from build123d import *

# Parameters (mm, degrees)
F0_W             = 150
F0_H             = 80
F1_DEPTH         = 8
F2_SIZE          = 2.5
F4_D             = 4.4
F4_COPIES_COUNT  = 4
F4_COPIES2_COUNT = 2
F4_COPIES2_PITCH = 104.737768
F4_COPIES3_COUNT = 2
F4_COPIES3_PITCH = 92.195445
F4_COPIES4_COUNT = 2
F4_COPIES4_PITCH = 67.720012
F5_D             = 6.5
F6_D             = 5.5
F7_D             = 29


# Not quite as in the source:
# - a pattern or mirror of a feature is missing from the dataset's text; its kind, count and spacing are read off the source's solid


with BuildPart() as f1:
    # F0 (on Front) → F1 (new body)
    with BuildSketch(Plane.XZ):
        Rectangle(F0_W, F0_H)
    extrude(amount=F1_DEPTH)

    # F2
    f2_edges = [f1.edges().sort_by_distance(p)[0] for p in [
        (75, -4, 40),
        (75, -4, -40),
        (-75, -4, 40),
        (-75, -4, -40),
    ]]
    chamfer(f2_edges, length=F2_SIZE)

    # F4 (through all)
    with Locations(Plane.XZ.offset(8)):
        with Locations((42, 34)):
            f4 = Hole(F4_D / 2)

    # F4_copies: F4 ×4 about axis
    f4_copies_axis = Axis((42, 0, 15), (0, 1, 0))
    for i in range(1, F4_COPIES_COUNT):
        add(f4.rotate(f4_copies_axis, i * 360 / F4_COPIES_COUNT), mode=Mode.SUBTRACT)

    # F4_copies1: F4 across plane
    add(f4.mirror(Plane(origin=(0, 0, 0), x_dir=(0, 0, -1), z_dir=(-1, 0, 0))), mode=Mode.SUBTRACT)

    # F4_copies2: F4 ×2
    with Locations(*[Vector(-0.9834083939, 0, -0.1814054319) * (i * F4_COPIES2_PITCH) for i in range(1, F4_COPIES2_COUNT)]):
        add(f4, mode=Mode.SUBTRACT)

    # F4_copies3: F4 ×2
    with Locations(*[Vector(-0.9111079228, 0, -0.4121678699) * (i * F4_COPIES3_PITCH) for i in range(1, F4_COPIES3_COUNT)]):
        add(f4, mode=Mode.SUBTRACT)

    # F4_copies4: F4 ×2
    with Locations(*[Vector(-0.9598344457, 0, -0.2805669918) * (i * F4_COPIES4_PITCH) for i in range(1, F4_COPIES4_COUNT)]):
        add(f4, mode=Mode.SUBTRACT)

    # F5 (through all)
    with Locations(Plane.XZ.offset(8)):
        with Locations((67.5, 32.5), (67.5, -32.5), (-67.5, -32.5), (-67.5, 32.5)):
            Hole(F5_D / 2)

    # F6 (through all)
    with Locations(Plane.XZ.offset(8)):
        with Locations((-8.25, -8.25), (8.25, -8.25), (8.25, 8.25), (-8.25, 8.25)):
            Hole(F6_D / 2)

    # F7 (through all)
    with Locations(Plane.XZ.offset(8)):
        with Locations((-42, 15), (42, 15)):
            Hole(F7_D / 2)


solid = f1.part
Source: CAD feature listing. Evaluate the final solid. Frame: model axes, mm. Coordinates: 2 decimals unless noted, no trailing zeros. Loops run counter-clockwise (first coordinate to the right, second up) from the corner with the lowest first, then second, coordinate; pieces in that order, holes last. Notation, with made-up numbers: (66.5, 80.5) -> (81.5, 80.5) arc R25 cw to (81.5, 97.5) -> close; hole circle Ø3 at (32, 74). An arc over 180 degrees is marked (long way). Answer in a Markdown table with one row per item. Add a question column.
Q1. Section D-D on z = 15. Return the cut outline in (x, y), and give its area (3 significant figures).
Q2. Section A-A on x = -67.5. Return the cut outline in (y, z), and give its area (3 significant figures).
Q3. Ray query, line 1 along Z through (x, y) = (-67.5, -5.5); line 2 along Z through (x, y) = (-8.25, -4); line 3 along X through (y, z) = (-2.5, 9.5). Return the intervals inside material, ascending.
Q4. Pull-direction query (Z, two-part tool) for faces 1 (the face through (-1, -4, -40)), 2 (the face through (-1, -8, 1)), 3 (the face through (70.079, -3.944, 30.522)), 4 (the face through (-1, -4, 40)); classes: pulls with the +Z half, pulls with the -Z half, needs draft (parallel to the pull), parting line crosses it, or undercut.
Q5. Section C-C on x = -31.5. Return the cut outline in (y, z), and give its area (3 significant figures).
Q6. Section B-B on z = -4. Return the cut outline in (x, y), and give its area (3 significant figures).
Q7. Contact query for a flat-ended pin moving along its axis: pin 1 Ø5.5 at (x, z) = (-42, -4) entering from -Y. Output: stop coordinate, or through.
Computed values:
| question | item | result |
|---|---|---|
| 1 | outline | (-75, -8) -> (-63.2, -8) -> (-63.2, 0) -> (-75, 0) -> close; (-58.8, -8) -> (-56.5, -8) -> (-56.5, 0) -> (-58.8, 0) -> close; (-27.5, -8) -> (-25.2, -8) -> (-25.2, 0) -> (-27.5, 0) -> close; (-20.8, -8) -> (20.8, -8) -> (20.8, 0) -> (-20.8, 0) -> close; (25.2, -8) -> (27.5, -8) -> (27.5, 0) -> (25.2, 0) -> close; (56.5, -8) -> (58.8, -8) -> (58.8, 0) -> (56.5, 0) -> close; (63.2, -8) -> (75, -8) -> (75, 0) -> (63.2, 0) -> close |
| 1 | area | 595 mm^2 |
| 2 | outline | (-8, -40) -> (0, -40) -> (0, -35.75) -> (-8, -35.75) -> close; (-8, -29.25) -> (0, -29.25) -> (0, 29.25) -> (-8, 29.25) -> close; (-8, 35.75) -> (0, 35.75) -> (0, 40) -> (-8, 40) -> close |
| 2 | area | 536 mm^2 |
| 3 | line 1 | z = -40 to -35.75, -29.25 to 29.25, 35.75 to 40 |
| 3 | line 2 | z = -40 to -11, -5.5 to 5.5, 11 to 40 |
| 3 | line 3 | x = -75 to -55.42, -28.58 to -10.7, -5.8 to 5.8, 10.7 to 28.58, 55.42 to 75 |
| 4 | face 1 | pulls with the -Z half |
| 4 | face 2 | needs draft |
| 4 | face 3 | undercut |
| 4 | face 4 | pulls with the +Z half |
| 5 | outline | (-8, -40) -> (0, -40) -> (0, 5) -> (-8, 5) -> close; (-8, 25) -> (0, 25) -> (0, 40) -> (-8, 40) -> close |
| 5 | area | 480 mm^2 |
| 6 | outline | (-75, -8) -> (-44.2, -8) -> (-44.2, 0) -> (-75, 0) -> close; (-39.8, -8) -> (39.8, -8) -> (39.8, 0) -> (-39.8, 0) -> close; (44.2, -8) -> (75, -8) -> (75, 0) -> (44.2, 0) -> close |
| 6 | area | 1,130 mm^2 |
| 7 | pin 1 | stops at y = -8 |
